```python
from build123d import *

# Parameters (mm, degrees)
F0_W       = 92.71
F0_H       = 73.66
F1_DEPTH   = 5.08
F2_W       = 92.71
F2_H       = 12.7
F3_DEPTH   = 20.32
F5_DEPTH   = 73.661
F6_SIZE2   = 1.111096
F6_SIZE    = 12.69999
F6_2_SIZE2 = 1.111096
F6_2_SIZE  = 12.69999


# Not quite as in the source:
# - a fillet or chamfer is up to 0.001 mm smaller than in the source, because OpenCascade refuses the exact size


with BuildPart() as f1:
    # F0 (on Top) → F1 (new body)
    with BuildSketch(Plane.XY):
        Rectangle(F0_W, F0_H)
    extrude(amount=F1_DEPTH)

    # F2 (on face) → F3 (join)
    with BuildSketch(Plane(origin=(0, 0, 0), x_dir=(1, 0, 0), z_dir=(0, 0, -1))):
        with Locations((0, 30.48)):
            Rectangle(F2_W, F2_H)
        with Locations((0, -30.48)):
            Rectangle(F2_W, F2_H)
    extrude(amount=F3_DEPTH)

    # F4 (on face) → F5 (cut, through all)
    with BuildSketch(Plane.XZ.offset(36.83)):
        with BuildLine():
            Line((-46.355, -20.32), (46.355, -20.32))
            ThreePointArc((46.355, -20.32), (0, -5.08), (-46.355, -20.32))
        make_face()
    extrude(amount=-F5_DEPTH, mode=Mode.SUBTRACT)

    # F6 (size 12.7 and 1.1111060268 in the source; OpenCascade refuses exactly that, so slightly less here)
    f6_edges = [f1.edges().sort_by_distance(p)[0] for p in [
        (0, 24.13, -5.08),
    ]]
    f6_side = f1.faces().sort_by_distance((0, 30.48, -5.08))[0]
    chamfer(f6_edges, length=F6_SIZE, length2=F6_SIZE2, reference=f6_side)

    # F6#2 (size 12.7 and 1.1111060268 in the source; OpenCascade refuses exactly that, so slightly less here)
    f6_2_edges = [f1.edges().sort_by_distance(p)[0] for p in [
        (0, -24.13, -5.08),
    ]]
    f6_2_side = f1.faces().sort_by_distance((0, -30.48, -5.08))[0]
    chamfer(f6_2_edges, length=F6_2_SIZE, length2=F6_2_SIZE2, reference=f6_2_side)


solid = f1.part
```
CAD build for the part. Positions are in the model's coordinates, mm. A direction names the side the tool comes from. Give positions to 0.01 mm unless a question says otherwise; leave off trailing zeros. Order: outer loops, then holes, each group sorted by start corner. A loop starts at its lowest first (then second) coordinate and runs counter-clockwise, first axis right, second up.
(1) Saw through at D-D, the plane y = -31. Give the cut face in (x, z) (3 decimals).
(2) Saw through at A-A, the plane y = -14. Give the cut face in (x, z) (3 decimals), then the cut area to 3 significant figures.
(3) Drill centre lines: L1, parallel to Y at x = 33.5, z = -3.5; L2, parallel to Z at x = -25, y = 18.5; L3, parallel to X at y = 33.5, z = -13 (3 decimals). Where is each one in solid material? Low to high.
(4) Mould opens along X. For faces 1 (the flat face through (-1, 36.83, -2)), 2 (the flat face through (-46.355, 9, 1)), 3 (the flat face through (46.355, 9, 1)), 4 (the conical face through (0.7, -30.39, -4.52)) say: released by +X, released by -X, zero draft, split by the parting line, or undercut.
(5) Saw through at B-B, the plane z = -6.5. State how many separate pieces and enclosed holes the cut face has, then the cut area to 3 significant figures.
(6) Tool access for faces 5 (the conical face through (0.7, 30.39, -4.52)), 6 (the flat face through (-1, 0, 0)), 7 (the flat face through (-1, -36.83, -2)): list every direction of +Z, -Z, +X, -X, +Y, -Y with a clear straight run to the whole face (end or side of a thin tool).
Results found:
1. outline: (-46.355, -19.687) arc R78.628 cw to (46.355, -19.687) - (46.355, 5.08) - (-46.355, 5.08) - close
2. outline: (-46.355, 0) - (46.355, 0) - (46.355, 5.08) - (-46.355, 5.08) - close
2. area: 471 mm2
3. L1: y = -36.83 to -24.13, 24.13 to 36.83
3. L2: z = 0 to 5.08
3. L3: x = -46.355 to -34.932, 34.932 to 46.355
4. face 1: zero draft
4. face 2: released by -X
4. face 3: released by +X
4. face 4: undercut
5. separate pieces: 4
5. enclosed holes: 0
5. area: 1,470 mm2
6. face 5: -Z
6. face 6: -Z, +X, -X
6. face 7: +Z, -Z, +X, -X, -Y
